```python
from build123d import *

# Parameters (mm, degrees)
SKETCH1_W           = 4.3
SKETCH1_H           = 1.399999994
BOSS_EXTRUDE1_DEPTH = 7.75
SKETCH2_W           = 7.2
SKETCH2_H           = 7.2
BOSS_EXTRUDE2_DEPTH = 2
FILLET1_R           = 1.25


with BuildPart() as part:
    # Sketch1 → Boss-Extrude1 (new body)
    with BuildSketch(Plane(origin=(0, 0, 0), x_dir=(1, 0, 0), z_dir=(0, 1, 0))):
        Rectangle(SKETCH1_W, SKETCH1_H)
    extrude(amount=BOSS_EXTRUDE1_DEPTH)

    # Sketch2 → Boss-Extrude2 (add)
    with BuildSketch(Plane(origin=(0, 7.75, 0), x_dir=(1, 0, 0), z_dir=(0, 1, 0))):
        Rectangle(SKETCH2_W, SKETCH2_H)
    extrude(amount=BOSS_EXTRUDE2_DEPTH)

    # Fillet1
    fillet1_edges = [part.edges().sort_by_distance(p)[0] for p in [
        (-2.15, 7.75, 0),
        (0, 7.75, 0.699999997),
        (2.15, 7.75, 0),
        (0, 7.75, -0.699999997),
    ]]
    fillet(fillet1_edges, radius=FILLET1_R)
    fillet1_2_edges = [part.edges().sort_by_distance(p)[0] for p in [
        (3.6, 8.75, 3.6),
        (3.6, 8.75, -3.6),
        (-3.6, 8.75, -3.6),
        (-3.6, 8.75, 3.6),
    ]]
    fillet(fillet1_2_edges, radius=FILLET1_R)


solid = part.part
```
Read the model definition and answer for the solid it produces. Units are mm, in the model's axes. A direction names the side the tool comes from. Round coordinates to 2 decimals unless told otherwise and drop trailing zeros. Write each loop counter-clockwise with the first axis right and the second up, starting at its lowest first coordinate (ties: lowest second). Pieces come first, ordered by that corner, then holes. Notation, with made-up numbers: (-24, 78) - (26, 78) arc R24 cw to (26, 93) - close; hole circle Ø5 at (6, -14.5). An arc over 180 degrees is marked (long way). One line per item, written item: value.
Q1. Which of the six approach directions +Z, -Z, +X, -X, +Y, -Y give full straight-line access (tool end or side, diameter ignored) to faces 1 (the flat face through (0, 3, -0.7)), 2 (the flat face through (2.15, 3, 0)), 3 (the cylindrical face through (-3.244, 8.764, -3.224)), 4 (the flat face through (-2.15, 3, 0))?
The answers:
face 1: -Z, +X, -X, -Y
face 2: +Z, -Z, +X, -Y
face 3: -Z, -X, +Y, -Y
face 4: +Z, -Z, -X, -Y
Q2. Find section A-A (z = -0.25). Determine the outline of the cut face in (x, y), and give its area (3 significant figures).
The answers:
outline: (-3.6, 7.75) - (-3.4, 7.75) arc R1.25 cw to (-2.15, 6.5) - (-2.15, 0) - (2.15, 0) - (2.15, 6.5) arc R1.25 cw to (3.4, 7.75) - (3.6, 7.75) - (3.6, 9.75) - (-3.6, 9.75) - close
area: 48.4 mm2
Q3. Find section D-D (x = -3). Determine the outline of the cut face in (y, z).
The answers:
outline: (7.68, -1.55) arc R1.25 cw to (7.75, -1.95) - (7.75, -3.42) - (9.75, -3.42) - (9.75, 3.42) - (7.75, 3.42) - (7.75, 1.95) arc R1.25 cw to (7.68, 1.55) - close
Q4. Straight lines are drawn through the part: line 1 (Y direction, x = -0.75, z = -2.5); line 2 (Z direction, x = 0.25, y = 3.5); line 3 (X direction, y = 3, z = 0.5). For each, find the intervals that lie inside material, in ascending order. Write a range as from..to.
The answers:
line 1: y = 7.75..9.75
line 2: z = -0.7..0.7
line 3: x = -2.15..2.15
Q5. Find section B-B (x = -1.5). Determine the outline of the cut face in (y, z).
The answers:
outline: (0, -0.7) - (6.5, -0.7) arc R1.25 cw to (7.75, -1.95) - (7.75, -3.6) - (9.75, -3.6) - (9.75, 3.6) - (7.75, 3.6) - (7.75, 1.95) arc R1.25 cw to (6.5, 0.7) - (0, 0.7) - close
Q6. Each of these flat-tipped pins is pushed along its axis until it touches: P1, Ø0.7, axis at y = 2.5, z = 0, coming from the -X side; P2, Ø1.3, axis at x = -0.5, y = 2.5, coming from the -Z side; P3, Ø1.1, axis at y = 2, z = 0, coming from the +X side. Where does it stop, or does it pass through?
The answers:
P1: stops at x = -2.15
P2: stops at z = -0.7
P3: stops at x = 2.15
Q7. Find section C-C (y = 2.25). Determine the outline of the cut face in (x, z), and give its area (3 significant figures).
The answers:
outline: (-2.15, -0.7) - (2.15, -0.7) - (2.15, 0.7) - (-2.15, 0.7) - close
area: 6.02 mm2
